Input: part model. Units: mm. Frame: model coordinates. A direction names the side the tool comes from. Give positions to 0.01 mm unless a question says otherwise; leave off trailing zeros. Loops run counter-clockwise (first coordinate to the right, second up) from the corner with the lowest first, then second, coordinate; pieces in that order, holes last. Notation, with made-up numbers: M 67,19 L 116,19 A12 cw 116,35 Z; hole C 42.25,-15 d4. An arc over 180 degrees is marked long. Answer as a JSON object with one key per item and string values. Group by question number.
```python
from build123d import *

# Parameters (mm, degrees)
SKETCH1_R           = 10
BOSS_EXTRUDE1_DEPTH = 30
BOSS_EXTRUDE2_DEPTH = 15


with BuildPart() as part:
    # Sketch1 → Boss-Extrude1 (new body, symmetric)
    with BuildSketch(Plane.XY):
        Circle(SKETCH1_R)
    boss_extrude1 = extrude(amount=BOSS_EXTRUDE1_DEPTH, both=True)

    # Sketch2 → Boss-Extrude2 (add, symmetric)
    with BuildSketch(Plane.XY):
        with BuildLine():
            Line((0, 20), (55, 20))
            Line((55, 20), (55, -20))
            Line((55, -20), (0, -20))
            ThreePointArc((0, -20), (-20, 0), (0, 20))
        make_face()
    boss_extrude2 = extrude(amount=BOSS_EXTRUDE2_DEPTH, both=True)

    # Mirror1: Boss-Extrude1, Boss-Extrude2 across plane
    add(boss_extrude1.mirror(Plane(origin=(55, 20, 15), x_dir=(0, 0, 1), z_dir=(-1, 0, 0))))
    add(boss_extrude2.mirror(Plane(origin=(55, 20, 15), x_dir=(0, 0, 1), z_dir=(-1, 0, 0))))


solid = part.part
```
1. First-contact query: P1, Ø20, axis at x = 87, y = 3.5, coming from the +Z side; P2, Ø6, axis at y = -4.5, z = 17.5, coming from the -X side; P3, Ø6, axis at x = 15.5, y = -0.5, coming from the -Z side; P4, Ø12, axis at x = 8, y = 8.5, coming from the +Z side. Flat tips, straight axial feed; report the tip coordinate or a pass-through.
2. Section D-D (x = 21). Output: boundary loops of the cut face in (y, z), then the cut area to 3 significant figures.
3. Material intervals for L1, parallel to Z at x = 95, y = 5; L2, parallel to X at y = 2, z = -20; L3, parallel to X at y = 3, z = 6, sorted ascending.
4. Section A-A (y = 0). Output: boundary loops of the cut face in (x, z).
5. Mould query, pull axis X, two halves, no side actions, for faces 4 (the cylindrical face through (-2.17, -9.76, 22.6)), 5 (the cylindrical face through (130, 0, 0)), 6 (the flat face through (0, 0, 30)). Classes: pulls with the +X half, pulls with the -X half, needs draft (parallel to the pull), parting line crosses it, or undercut.
6. Reachability of faces 1 (the flat face through (54, -20, 0)), 2 (the cylindrical face through (120, 0, -22)), 3 (the cylindrical face through (120, 0, 23)) from +Z, -Z, +X, -X, +Y, -Y: full face, straight path, thin tool, end or side. Return the list, or none.
7. Section B-B (z = -26). Output: boundary loops of the cut face in (x, y), then the cut area to 3 significant figures.
8. Section C-C (z = 9.5). Output: boundary loops of the cut face in (x, y).
Geometry results:
{
 "1": {"P1": "z = 15", "P2": "x = -19.8", "P3": "z = -15", "P4": "z = 30"},
 "2": {"outline": "M -20,-15 L 20,-15 L 20,15 L -20,15 Z", "area": "1,200 mm2"},
 "3": {"L1": "-15 to 15", "L2": "-9.8 to 9.8, 100.2 to 119.8", "L3": "-19.77 to 129.77"},
 "4": {"outline": "M -20,-15 L -10,-15 L -10,-30 L 10,-30 L 10,-15 L 100,-15 L 100,-30 L 120,-30 L 120,-15 L 130,-15 L 130,15 L 120,15 L 120,30 L 100,30 L 100,15 L 10,15 L 10,30 L -10,30 L -10,15 L -20,15 Z"},
 "5": {"face 4": "undercut", "face 5": "pulls with the +X half", "face 6": "needs draft"},
 "6": {"face 1": "+Z, -Z, +X, -X, -Y", "face 2": "-Z", "face 3": "+Z"},
 "7": {"outline": "C 0,0 d20; C 110,0 d20", "area": "628 mm2"},
 "8": {"outline": "M 0,-20 L 110,-20 A20 ccw 110,20 L 0,20 A20 ccw Z"}
}
